```python
from build123d import *

# Parameters (mm, degrees)
F0_W        = 26.5
F0_H        = 19
F1_DEPTH    = 2
F2_DEPTH    = 8
F3_T1_DEPTH = 23
F3_T3_DEPTH = 11.1067326603
F3_T5_DEPTH = 28


# Not quite as in the source:
# - a fillet or chamfer that OpenCascade refuses, or shapes differently, is made with other operations: its cross-section is extruded or revolved along the edge and cut away or added


with BuildPart() as f1:
    # F0 (on Top) → F1 (new body)
    with BuildSketch(Plane.XY):
        Polygon((-5.2328903973, 8.0285165012), (-35.2328903973, 8.0285165012), (-35.2328903973, -14.9714834988), (-5.2328903973, -14.9714834988), (-5.2328903973, -13.9714834988), (-5.2328903973, -11.9714834988), (-5.2328903973, 5.0285165012), (-5.2328903973, 7.0285165012), align=None)
        with Locations((-19.9828903973, -3.4714834988)):
            Rectangle(F0_W, F0_H, mode=Mode.SUBTRACT)
        Polygon((-2.8519380164, 5.0285165012), (-5.2328903973, 7.0285165012), (-5.2328903973, 5.0285165012), align=None)
        Polygon((-2.1233994035, 7.0285165012), (-5.2328903973, 7.0285165012), (-2.8519380164, 5.0285165012), (0.2575529774, 5.0285165012), align=None)
        Polygon((0.2575529774, 5.0285165012), (-2.8519380164, 5.0285165012), (7.2671096027, -3.4714834988), (8.8218550996, -2.1654972814), align=None)
        Polygon((-5.2328903973, -11.9714834988), (-5.2328903973, -13.9714834988), (-2.8519380164, -11.9714834988), align=None)
        Polygon((-2.8519380164, -11.9714834988), (-5.2328903973, -13.9714834988), (-2.1233994035, -13.9714834988), (0.2575529774, -11.9714834988), align=None)
        Polygon((8.8218550996, -4.7774697162), (7.2671096027, -3.4714834988), (-2.8519380164, -11.9714834988), (0.2575529774, -11.9714834988), align=None)
        Polygon((8.8218550996, -2.1654972814), (7.2671096027, -3.4714834988), (8.8218550996, -4.7774697162), (10.3766005965, -3.4714834988), align=None)
        Polygon((21.3218550996, 5.7225302838), (19.7671096027, 7.0285165012), (8.8218550996, -2.1654972814), (10.3766005965, -3.4714834988), (19.7671096027, 4.4165440664), align=None)
        Polygon((10.3766005965, -3.4714834988), (8.8218550996, -4.7774697162), (19.7671096027, -13.9714834988), (21.3218550996, -12.6654972814), (19.7671096027, -11.359511064), align=None)
        Polygon((19.7671096027, -11.359511064), (21.3218550996, -12.6654972814), (30.7123641058, -4.7774697162), (29.1576186089, -3.4714834988), align=None)
        Polygon((30.7123641058, -2.1654972814), (21.3218550996, 5.7225302838), (19.7671096027, 4.4165440664), (29.1576186089, -3.4714834988), align=None)
        Polygon((32.2671096027, -3.4714834988), (30.7123641058, -2.1654972814), (29.1576186089, -3.4714834988), (30.7123641058, -4.7774697162), align=None)
        Polygon((41.7671096027, 7.0285165012), (41.6576186089, 7.0285165012), (30.7123641058, -2.1654972814), (32.2671096027, -3.4714834988), (41.7671096027, 4.5085165012), align=None)
        Polygon((30.7123641058, -4.7774697162), (41.6576186089, -13.9714834988), (41.7671096027, -13.9714834988), (41.7671096027, -11.4514834988), (32.2671096027, -3.4714834988), align=None)
    extrude(amount=F1_DEPTH)

    # F0 (on Top) → F2 (join)
    with BuildSketch(Plane.XY):
        Polygon((44.7671096027, 7.0285165012), (41.7671096027, 7.0285165012), (41.7671096027, 4.5085165012), align=None)
        Polygon((44.7671096027, 7.0285165012), (41.7671096027, 4.5085165012), (41.7671096027, -11.4514834988), (44.7671096027, -13.9714834988), align=None)
        Polygon((41.7671096027, -11.4514834988), (41.7671096027, -13.9714834988), (44.7671096027, -13.9714834988), align=None)
    extrude(amount=F2_DEPTH)

    # F3: fillet of radius 5 on 8 edges, made by hand

    # F3_s2 → F3_t1 (cut)
    with BuildSketch(Plane.XY.offset(-10.5)):
        with BuildLine():
            ThreePointArc((22.9830700348, -11.2700767358), (19.7671096027, -12.4415524119), (16.5511491706, -11.2700767358))
            Line((16.5511491706, -11.2700767358), (19.7671096027, -13.9714834988))
            Line((19.7671096027, -13.9714834988), (22.9830700348, -11.2700767358))
        make_face()
        with BuildLine():
            ThreePointArc((16.5511491706, 4.3271097382), (19.7671096027, 5.4985854143), (22.9830700348, 4.3271097382))
            Line((22.9830700348, 4.3271097382), (19.7671096027, 7.0285165012))
            Line((19.7671096027, 7.0285165012), (16.5511491706, 4.3271097382))
        make_face()
    extrude(amount=F3_T1_DEPTH, mode=Mode.SUBTRACT)

    # F3_s4 → F3_t3 (cut)
    with BuildSketch(Plane.XY.offset(-4.5533663301)):
        with BuildLine():
            ThreePointArc((-0.7287855035, -12.8000078228), (-2.2334045932, -13.6694948664), (-3.9447459356, -13.9714834988))
            Line((-3.9447459356, -13.9714834988), (-2.1233994035, -13.9714834988))
            Line((-2.1233994035, -13.9714834988), (-0.7287855035, -12.8000078228))
        make_face()
        with BuildLine():
            ThreePointArc((-3.9447459356, 7.0285165012), (-2.2334045932, 6.7265278688), (-0.7287855035, 5.8570408251))
            Line((-0.7287855035, 5.8570408251), (-2.1233994035, 7.0285165012))
            Line((-2.1233994035, 7.0285165012), (-3.9447459356, 7.0285165012))
        make_face()
        with BuildLine():
            ThreePointArc((40.2630047089, 5.8570408251), (41.7676237986, 6.7265278688), (43.478965141, 7.0285165012))
            Line((43.478965141, 7.0285165012), (41.6576186089, 7.0285165012))
            Line((41.6576186089, 7.0285165012), (40.2630047089, 5.8570408251))
        make_face()
        with BuildLine():
            ThreePointArc((43.478965141, -13.9714834988), (41.7676237986, -13.6694948664), (40.2630047089, -12.8000078228))
            Line((40.2630047089, -12.8000078228), (41.6576186089, -13.9714834988))
            Line((41.6576186089, -13.9714834988), (43.478965141, -13.9714834988))
        make_face()
    extrude(amount=F3_T3_DEPTH, mode=Mode.SUBTRACT)

    # F3_s6 → F3_t5 (cut)
    with BuildSketch(Plane.YZ.offset(29.2671096027)):
        with BuildLine():
            ThreePointArc((-8.9714834988, 8), (-12.5070174047, 6.5355339059), (-13.9714834988, 3))
            Line((-13.9714834988, 3), (-13.9714834988, 8))
            Line((-13.9714834988, 8), (-8.9714834988, 8))
        make_face()
        with BuildLine():
            ThreePointArc((7.0285165012, 3), (5.5640504071, 6.5355339059), (2.0285165012, 8))
            Line((2.0285165012, 8), (7.0285165012, 8))
            Line((7.0285165012, 8), (7.0285165012, 3))
        make_face()
    extrude(amount=F3_T5_DEPTH, mode=Mode.SUBTRACT)


solid = f1.part
```
For this review, take the finished solid that the model builds, in its own axes (mm). A direction names the side the tool comes from. Coordinates: 2 decimals unless noted, no trailing zeros. Order: outer loops, then holes, each group sorted by start corner. A loop starts at its lowest first (then second) coordinate and runs counter-clockwise, first axis right, second up. Notation, with made-up numbers: (-9.75, -31.5) - (15.25, -31.5) arc R11 ccw to (15.25, -18.5) - close; hole circle Ø6 at (15, 66.25). An arc over 180 degrees is marked (long way). Answer as a JSON object with one key per item and string values. Group by question number.
1. Clearance check with flat-ended pins moving along their axes: P1, Ø1.4, axis at x = -4.5, z = 1.5, coming from the -Y side; P2, Ø3, axis at x = -21, z = 4.5, coming from the -Y side; P3, Ø4, axis at y = -0.5, z = 5.5, coming from the -X side; P4, Ø4, axis at x = 10, y = -4.5, coming from the +Z side. State where each tip first meets the part, or that it passes through.
2. For probe 1 along X at (y, z) = (-3.25, 1); probe 2 along Z at (x, y) = (15, -9.25); probe 3 along X at (y, z) = (-8.5, 4.5), list the stretches that pass through material, from the lowest coordinate up.
3. We need section B-B on y = 3. State the section outline as (x, z) points.
4. The part is to be moulded in two halves that separate along X. For faces 4 (the flat face through (-35.233, -3, 1)), 5 (the flat face through (-5, 7.029, 1)), 6 (the flat face through (-20, -12.971, 1)), 7 (the flat face through (44.767, -4, 4)), say which applies: pulls with the +X half, pulls with the -X half, needs draft (parallel to the pull), parting line crosses it, or undercut.
5. We need section A-A on x = -10. State the section outline as (y, z) points.
6. We need section D-D on z = 1.25. Give the number of separate pieces and of enclosed holes in the cut face, then the cut area to 3 significant figures.
7. We need section C-C on x = 28. State the section outline as (y, z) points.
8. For faces 1 (the flat face through (44, -13.971, 1)), 2 (the flat face through (41.767, -3, 4)), 3 (the flat face through (-5.233, -4, 1)), list the 3-axis set-ups (+Z, -Z, +X, -X, +Y, -Y) from which the entire face can be reached by the end or side of a thin tool; tool diameter is ignored.
Final values:
{
 "1": {"P1": "y = -13.97", "P2": "through", "P3": "x = 41.77", "P4": "z = 2"},
 "2": {"probe 1": "-35.23 to -33.23, -6.73 to -5.23, 7 to 10.64, 28.89 to 32.53, 41.77 to 44.77", "probe 2": "0 to 2", "probe 3": "41.77 to 44.77"},
 "3": {"outline": "(-35.23, 0) - (-33.23, 0) - (-33.23, 2) - (-35.23, 2) - close; (-6.73, 0) - (-5.23, 0) - (-5.23, 2) - (-6.73, 2) - close; (-0.44, 0) - (2.67, 0) - (2.67, 2) - (-0.44, 2) - close; (14.97, 0) - (18.08, 0) - (18.08, 2) - (14.97, 2) - close; (21.45, 0) - (24.56, 0) - (24.56, 2) - (21.45, 2) - close; (36.86, 0) - (39.97, 0) - (39.97, 2) - (36.86, 2) - close; (41.77, 0) - (44.77, 0) - (44.77, 7.9) - (41.77, 7.9) - close"},
 "4": {"face 4": "pulls with the -X half", "face 5": "needs draft", "face 6": "undercut", "face 7": "pulls with the +X half"},
 "5": {"outline": "(-14.97, 0) - (-12.97, 0) - (-12.97, 2) - (-14.97, 2) - close; (6.03, 0) - (8.03, 0) - (8.03, 2) - (6.03, 2) - close"},
 "6": {"separate pieces": "1", "enclosed holes": "4", "area": "475 mm²"},
 "7": {"outline": "(-7.06, 0) - (-4.44, 0) - (-4.44, 2) - (-7.06, 2) - close; (-2.5, 0) - (0.11, 0) - (0.11, 2) - (-2.5, 2) - close"},
 "8": {"face 1": "+Z, -Z, +X, -Y", "face 2": "+Z", "face 3": "+Z, -Z"}
}
